from build123d import *

# Parameters (mm, degrees)
SKETCH1_R                      = 3.5
SKETCH1_R_2                    = 1.5
BOSS_EXTRUDE1_DEPTH            = 8
CUT_EXTRUDE1_REACH             = 11.407
SKETCH2_R                      = 0.5
CUT_EXTRUDE1_DIRECTION_2_REACH = 11.407
SKETCH3_R                      = 0.5
CUT_EXTRUDE2_DEPTH             = 3.5
CUT_EXTRUDE3_START             = 4
SKETCH4_R                      = 0.6
CUT_EXTRUDE3_DEPTH             = 1
CUT_EXTRUDE4_START             = 4
SKETCH7_R                      = 0.6
CUT_EXTRUDE4_DEPTH             = 1


with BuildPart() as part:
    # Sketch1 → Boss-Extrude1 (new body)
    with BuildSketch(Plane(origin=(0, 0, 0), x_dir=(1, 0, 0), z_dir=(0, 1, 0))):
        with Locations(Location((0, 0, 0), (0, 0, 270))):
            Circle(SKETCH1_R)
        with Locations(Location((0, 0, 0), (0, 0, 270))):
            Circle(SKETCH1_R_2, mode=Mode.SUBTRACT)
    extrude(amount=BOSS_EXTRUDE1_DEPTH)

    # Sketch2 → Cut-Extrude1 (cut, up to next)
    with BuildSketch(Plane(origin=(0, 0, 0), x_dir=(0, 0, -1), z_dir=(1, 0, 0)), mode=Mode.PRIVATE) as cut_extrude1_sk1:
        with Locations((0, 5)):
            Circle(SKETCH2_R)
    cut_extrude1_tool1 = extrude(cut_extrude1_sk1.sketch, amount=-CUT_EXTRUDE1_REACH, mode=Mode.PRIVATE) & part.part
    add(cut_extrude1_tool1.solids().sort_by_distance((0, 5, 0))[0], mode=Mode.SUBTRACT)

    # Sketch2 → Cut-Extrude1 direction 2 (cut, up to next)
    with BuildSketch(Plane(origin=(0, 0, 0), x_dir=(0, 0, -1), z_dir=(1, 0, 0)), mode=Mode.PRIVATE) as cut_extrude1_direction_2_sk1:
        with Locations((0, 5)):
            Circle(SKETCH2_R)
    cut_extrude1_direction_2_tool1 = extrude(cut_extrude1_direction_2_sk1.sketch, amount=CUT_EXTRUDE1_DIRECTION_2_REACH, mode=Mode.PRIVATE) & part.part
    add(cut_extrude1_direction_2_tool1.solids().sort_by_distance((0, 5, 0))[0], mode=Mode.SUBTRACT)

    # Sketch3 → Cut-Extrude2 (cut, symmetric)
    with BuildSketch(Plane.XY):
        with Locations((0, 2)):
            Circle(SKETCH3_R)
    extrude(amount=CUT_EXTRUDE2_DEPTH, both=True, mode=Mode.SUBTRACT)

    # Sketch4 → Cut-Extrude3 (cut)
    with BuildSketch(Plane.XY.offset(CUT_EXTRUDE3_START)):
        with Locations((0, 2)):
            Circle(SKETCH4_R)
    extrude(amount=-CUT_EXTRUDE3_DEPTH, mode=Mode.SUBTRACT)

    # Sketch7 → Cut-Extrude4 (cut)
    with BuildSketch(Plane(origin=(0, 0, 0), x_dir=(0, 0, -1), z_dir=(1, 0, 0)).offset(CUT_EXTRUDE4_START)):
        with Locations((0, 5)):
            Circle(SKETCH7_R)
    extrude(amount=-CUT_EXTRUDE4_DEPTH, mode=Mode.SUBTRACT)


solid = part.part
The model under review builds one solid part; all positions refer to its coordinate system, in mm. A direction names the side the tool comes from. Give positions to 0.01 mm unless a question says otherwise; leave off trailing zeros. Write each loop counter-clockwise with the first axis right and the second up, starting at its lowest first coordinate (ties: lowest second). Pieces come first, ordered by that corner, then holes.
1. Add section A-A, the plane x = 0. Write out the cut boundary in (y, z), plus the area to 3 significant figures.
2. Add section B-B, the plane z = 0. Write out the cut boundary in (x, y).
3. Tool access review of faces 1 (the flat face through (0, 8, 2)), 2 (the cylindrical face through (3.254, 4.77, -0.554)), 3 (the cylindrical face through (0.572, 2.18, 3.254)): name each direction out of +Z, -Z, +X, -X, +Y, -Y from which nothing blocks a thin tool from reaching the whole face with its end or side.
4. Add section D-D, the plane y = 2. Write out the cut boundary in (x, z).
5. For P1, Ø3, axis at y = 3, z = 2, coming from the -X side; P2, Ø1, axis at x = -1.5, y = 3.5, coming from the +Z side; P3, Ø0.6, axis at y = 5, z = -0.5, coming from the +X side, all flat-tipped, find the tip position at first contact; note any pin that passes through.
6. Add section C-C, the plane x = 1. Write out the cut boundary in (y, z), plus the area to 3 significant figures.
7. Wall thickness on L1, parallel to Z at x = 0, y = 2.75; L2, parallel to Y at x = 0, z = 2.4; L3, parallel to Y at x = 2.35, z = 0: over which ranges is each line inside the solid? List them lowest first.
8. Draft analysis for pull direction X (two halves, no side actions). For faces 4 (the cylindrical face through (-1.341, 3.944, 3.233)), 5 (the cylindrical face through (2.196, 5.15, -0.477)), 6 (the cylindrical face through (-0.065, 2.496, -2.443)), state which applies: +X half, -X half, draft (parallel to the pull), parting line (faces both ways), or undercut.
Worked answers:
1. outline: (0, -3.5) - (1.5, -3.5) - (1.5, -1.5) - (0, -1.5) - close; (0, 1.5) - (1.5, 1.5) - (1.5, 3) - (1.4, 3) - (1.4, 3.5) - (0, 3.5) - close; (2.5, -3.5) - (8, -3.5) - (8, -1.5) - (2.5, -1.5) - close; (2.5, 1.5) - (8, 1.5) - (8, 3.5) - (2.6, 3.5) - (2.6, 3) - (2.5, 3) - close
1. area: 27.9 mm2
2. outline: (-3.5, 0) - (-1.5, 0) - (-1.5, 4.5) - (-3.5, 4.5) - close; (-3.5, 5.5) - (-1.5, 5.5) - (-1.5, 8) - (-3.5, 8) - close; (1.5, 0) - (3.5, 0) - (3.5, 4.4) - (3, 4.4) - (3, 4.5) - (1.5, 4.5) - close; (1.5, 5.5) - (3, 5.5) - (3, 5.6) - (3.5, 5.6) - (3.5, 8) - (1.5, 8) - close
3. face 1: +Z, -Z, +X, -X, +Y
3. face 2: +X
3. face 3: +Z
4. outline: (-0.6, 3) - (-0.6, 3.45) arc R3.5 ccw to (-0.5, -3.46) - (-0.5, -1.41) arc R1.5 cw to (-0.5, 1.41) - (-0.5, 3) - close; (0.5, -3.46) arc R3.5 ccw to (0.6, 3.45) - (0.6, 3) - (0.5, 3) - (0.5, 1.41) arc R1.5 cw to (0.5, -1.41) - close
5. P1: stops at x = -3.46
5. P2: stops at z = 3.35
5. P3: stops at x = 3.46
6. outline: (0, -3.35) - (8, -3.35) - (8, -1.12) - (0, -1.12) - close; (0, 1.12) - (8, 1.12) - (8, 3.35) - (0, 3.35) - close
6. area: 35.8 mm2
7. L1: z = -3.5 to -1.5, 1.5 to 3.5
7. L2: y = 0 to 1.5, 2.5 to 8
7. L3: y = 0 to 4.5, 5.5 to 8
8. face 4: parting line
8. face 5: draft
8. face 6: undercut
